Design review of the part built by this model. Coordinates are the model's own, in mm. A direction names the side the tool comes from. Give positions to 0.01 mm unless a question says otherwise; leave off trailing zeros. Loops run counter-clockwise (first coordinate to the right, second up) from the corner with the lowest first, then second, coordinate; pieces in that order, holes last. Notation, with made-up numbers: M -11.5,80 L 40.5,80 A10 cw 40.5,94 Z; hole C 84,24 d3. An arc over 180 degrees is marked long. Use one line per item in the form item = value. Start each with the question number.
from build123d import *

# Parameters (mm, degrees)
BOSS_EXTRUDE1_DEPTH = 15
SKETCH2_R           = 1.6
BOSS_EXTRUDE2_DEPTH = 15


with BuildPart() as part:
    # Sketch1 → Boss-Extrude1 (new body)
    with BuildSketch(Plane(origin=(0, 0, 0), x_dir=(1, 0, 0), z_dir=(0, 1, 0))):
        with BuildLine():
            ThreePointArc((16.84, -62.837627462), (0, -65.055), (-16.84, -62.837627462))
            Line((-16.84, -62.837627462), (-16.84, -78.263768278))
            ThreePointArc((-16.84, -78.263768278), (0, -80.055), (16.84, -78.263768278))
            Line((16.84, -78.263768278), (16.84, -62.837627462))
        make_face()
    extrude(amount=BOSS_EXTRUDE1_DEPTH)

    # Sketch2 → Boss-Extrude2 (add)
    # profile 1 of 2: a face of its own
    with BuildSketch(Plane(origin=(0, 15, 0), x_dir=(1, 0, 0), z_dir=(0, 1, 0))):
        Polygon((-16.84, -62.837627462), (-84.997835254, -44.574790547), (-84.997835254, -58.000931363), (-67.997835254, -58.000931363), (-67.997835254, -64.556067635), (-16.84, -78.263768278), align=None)
        with Locations(Location((-24.335670508, -68.54223901, 0), (0, 0, 270))):
            Circle(SKETCH2_R, mode=Mode.SUBTRACT)
        with Locations(Location((-77.497835254, -54.297479899, 0), (0, 0, 270))):
            Circle(SKETCH2_R, mode=Mode.SUBTRACT)
    # profile 2 of 2: a face of its own
    with BuildSketch(Plane(origin=(0, 15, 0), x_dir=(1, 0, 0), z_dir=(0, 1, 0))):
        Polygon((84.997835254, -44.574790547), (16.84, -62.837627462), (16.84, -78.263768278), (67.997835254, -64.556067635), (67.997835254, -58.000931363), (84.997835254, -58.000931363), align=None)
        with Locations(Location((24.335670508, -68.54223901, 0), (0, 0, 270))):
            Circle(SKETCH2_R, mode=Mode.SUBTRACT)
        with Locations(Location((77.497835254, -54.297479899, 0), (0, 0, 270))):
            Circle(SKETCH2_R, mode=Mode.SUBTRACT)
    extrude(amount=-BOSS_EXTRUDE2_DEPTH)


solid = part.part
Q1. Take a section at B-B on y = 13. Give the boundary of the cut face in (x, z) (3 decimals), plus the area to 3 significant figures.
Q2. Clearance check with flat-ended pins moving along their axes: pin 1 Ø3.5 at (y, z) = (5.5, 62.5) entering from +X; pin 2 Ø4.5 at (x, y) = (-78, 11) entering from +Z; pin 3 Ø1 at (x, y) = (-60.5, 5) entering from -Z (3 decimals). State where each tip first meets the part, or that it passes through.
Q3. Take a section at C-C on z = 68.5. Give the boundary of the cut face in (x, y).
Q4. Wall thickness on probe 1 along Z at (x, y) = (-2, 4.25); probe 2 along Z at (x, y) = (-24, 1); probe 3 along Z at (x, y) = (-23, 6.5): over which ranges is each line inside the solid? List them lowest first.
Q5. The part is to be moulded in two halves that separate along Z. For faces 4 (the flat face through (-1, 0, 66)), 5 (the cylindrical face through (-75.91, 7.6, 54.09)), 6 (the flat face through (76, 8, 58.001)), say which applies: pulls with the +Z half, pulls with the -Z half, needs draft (parallel to the pull), parting line crosses it, or undercut.
Q6. For faces 1 (the flat face through (-50.442, 7.605, 53.834)), 2 (the flat face through (67.998, 8, 61)), 3 (the flat face through (-77, 8, 58.001)), list the 3-axis set-ups (+Z, -Z, +X, -X, +Y, -Y) from which the entire face can be reached by the end or side of a thin tool; tool diameter is ignored.
Q7. Take a section at D-D on x = 70. Give the boundary of the cut face in (y, z), plus the area to 3 significant figures.
Q8. Take a section at A-A on z = 60. Give the boundary of the cut face in (x, y).
Response values:
q1.outline = M -84.998,44.575 L -16.84,62.838 A65.055 cw 16.84,62.838 L 84.998,44.575 L 84.998,58.001 L 67.998,58.001 L 67.998,64.556 L 16.84,78.264 A80.055 ccw -16.84,78.264 L -67.998,64.556 L -67.998,58.001 L -84.998,58.001 Z; hole C -77.498,54.297 d3.2; hole C -24.336,68.542 d3.2; hole C 24.336,68.542 d3.2; hole C 77.498,54.297 d3.2
q1.area = 2,440 mm^2
q2.pin_1 = 68
q2.pin_2 = 58
q2.pin_3 = 51.005
q3.outline = M -53.28,0 L -25.94,0 L -25.94,15 L -53.28,15 Z; M -22.74,0 L 22.74,0 L 22.74,15 L -22.74,15 Z; M 25.94,0 L 53.28,0 L 53.28,15 L 25.94,15 Z
q4.probe_1 = 65.02 to 80.03
q4.probe_2 = 60.92 to 66.98, 70.11 to 76.35
q4.probe_3 = 61.19 to 67.66, 69.42 to 76.61
q5.face_4 = needs draft
q5.face_5 = undercut
q5.face_6 = pulls with the +Z half
q6.face_1 = -Z, +Y, -Y
q6.face_2 = +Z, +X, +Y, -Y
q6.face_3 = +Z, -X, +Y, -Y
q7.outline = M 0,48.59 L 15,48.59 L 15,58 L 0,58 Z
q7.area = 141 mm^2
q8.outline = M -68,0 L -27.43,0 L -27.43,15 L -68,15 Z; M 27.43,0 L 68,0 L 68,15 L 27.43,15 Z
